The model under review builds one solid part; all positions refer to its coordinate system, in mm. Coordinates: 2 decimals unless noted, no trailing zeros. Loops run counter-clockwise (first coordinate to the right, second up) from the corner with the lowest first, then second, coordinate; pieces in that order, holes last. Notation, with made-up numbers: M 46.5,2 L 90.5,2 A7 ccw 90.5,10 Z; hole C 1,10.25 d8. An arc over 180 degrees is marked long. Write item = value, one per line. Start each with the question number.
Q1. Clearance check with flat-ended pins moving along their axes: pin 1 Ø1.5 at (y, z) = (-34, 1.5) entering from +X; pin 2 Ø1.5 at (y, z) = (54.5, 1.5) entering from +X; pin 3 Ø1.5 at (y, z) = (-62, 1) entering from -X. State where each tip first meets the part, or that it passes through.
Q2. We need section A-A on z = 1.45. Count the separate pieces of the cut face and the enclosed holes in it, and give its area (3 significant figures).
Q3. We need section B-B on y = 6. Give the boundary of the cut face in (x, z).
Q4. Wall thickness on probe 1 along Y at (x, z) = (0, 2); probe 2 along X at (y, z) = (-88, 0.7); probe 3 along X at (y, z) = (-68.25, 0.65): over which ranges is each line inside the solid? List them lowest first.
from build123d import *

# Parameters (mm, degrees)
F0_R     = 1.5
F1_DEPTH = 3
F2_W     = 41.530054
F2_H     = 123.730924
F3_DEPTH = 3
F4_R     = 5


with BuildPart() as f1:
    # F0 (on Top) → F1 (new body)
    with BuildSketch(Plane.XY):
        Polygon((32, 99.771135), (-32, 99.771135), (-39.425235, 86), (-18.486274, 70.8194), (-18.486274, 41.134663), (-39.425235, 27.363142), (-35.128705, 16.014801), (-35.128705, -94.051212), (35.128705, -94.051212), (35.128705, -88.935837), (24.525635, -88.935837), (24.525635, -50.918393), (35.128705, -50.918393), (35.128705, 16.014801), (39.425235, 27.363142), (18.486274, 41.134663), (18.486274, 70.8194), (39.425235, 86), align=None)
        with BuildLine():
            ThreePointArc((-20, -86.5), (-18.93934, -86.93934), (-18.5, -88))
            ThreePointArc((-18.5, -88), (-21.06066, -89.06066), (-20, -86.5))
        make_face(mode=Mode.SUBTRACT)
        with BuildLine():
            ThreePointArc((-18.5, -68.25), (-18.93934, -69.31066), (-20, -69.75))
            ThreePointArc((-20, -69.75), (-21.06066, -67.18934), (-18.5, -68.25))
        make_face(mode=Mode.SUBTRACT)
        with BuildLine():
            ThreePointArc((-1.5, -88), (0, -86.5), (1.5, -88))
            ThreePointArc((1.5, -88), (0, -89.5), (-1.5, -88))
        make_face(mode=Mode.SUBTRACT)
        with BuildLine():
            ThreePointArc((21.5, -88), (20, -89.5), (18.5, -88))
            ThreePointArc((18.5, -88), (18.93934, -86.93934), (20, -86.5))
            ThreePointArc((20, -86.5), (21.06066, -86.93934), (21.5, -88))
        make_face(mode=Mode.SUBTRACT)
        with BuildLine():
            ThreePointArc((21.5, -68.25), (21.06066, -69.31066), (20, -69.75))
            ThreePointArc((20, -69.75), (18.93934, -67.18934), (21.5, -68.25))
        make_face(mode=Mode.SUBTRACT)
        with Locations((-32, 86)):
            Circle(F0_R, mode=Mode.SUBTRACT)
        with Locations((-20, 95)):
            Circle(F0_R, mode=Mode.SUBTRACT)
        with Locations((0, 95)):
            Circle(F0_R, mode=Mode.SUBTRACT)
        with Locations((20, 95)):
            Circle(F0_R, mode=Mode.SUBTRACT)
        with Locations((32, 86)):
            Circle(F0_R, mode=Mode.SUBTRACT)
    extrude(amount=F1_DEPTH)

    # F2 (on Top) → F3 (join)
    with BuildSketch(Plane.XY):
        with Locations((0.572829, -0.729354)):
            Rectangle(F2_W, F2_H)
    extrude(amount=F3_DEPTH)

    # F4
    f4_edges = [f1.edges().sort_by_distance(p)[0] for p in [
        (39.425235, 86, 1.5),
        (32, 99.771135, 1.5),
        (-32, 99.771135, 1.5),
        (-39.425235, 86, 1.5),
    ]]
    fillet(f4_edges, radius=F4_R)


solid = f1.part
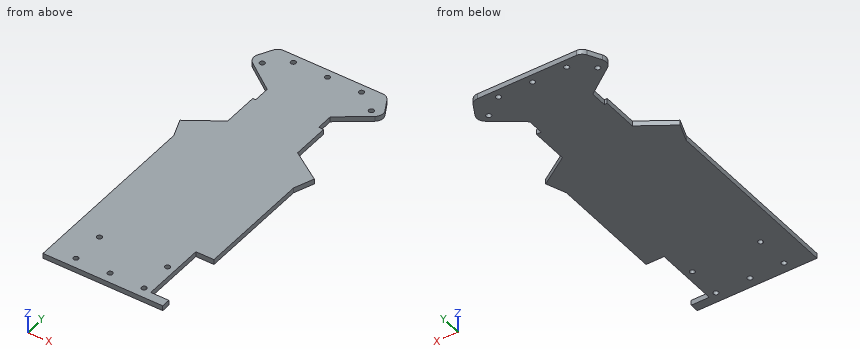
Returned:
q1.pin_1 = 35.13
q1.pin_2 = 21.34
q1.pin_3 = -35.13
q2.separate_pieces = 1
q2.enclosed_holes = 10
q2.area = 11,900 mm^2
q3.outline = M -35.13,0 L 35.13,0 L 35.13,3 L -35.13,3 Z
q4.probe_1 = -94.05 to -89.5, -86.5 to 93.5, 96.5 to 99.77
q4.probe_2 = -35.13 to -21.5, -18.5 to -1.5, 1.5 to 18.5, 21.5 to 24.53
q4.probe_3 = -35.13 to -21.5, -18.5 to 18.5, 21.5 to 24.53
